Source: CAD feature listing. Evaluate the final solid. Frame: model axes, mm. Round coordinates to 2 decimals unless told otherwise and drop trailing zeros. Write each loop counter-clockwise with the first axis right and the second up, starting at its lowest first coordinate (ties: lowest second). Pieces come first, ordered by that corner, then holes.
from build123d import *

# Parameters (mm, degrees)
BOSS_EXTRUDE1_DEPTH = 3.175
SKETCH2_W           = 2.286
SKETCH2_H           = 69.616100292
BOSS_EXTRUDE2_DEPTH = 3.175
FILLET1_R           = 1


with BuildPart() as part:
    # Sketch1 → Boss-Extrude1 (new body)
    with BuildSketch(Plane(origin=(0, 0, 0), x_dir=(1, 0, 0), z_dir=(0, 1, 0))):
        Polygon((83.6803, 0), (96.3803, 0), (96.3803, 143.6878), (0, 143.6878), (0, 0), (12.7, 0), (12.7, -2.286), (83.6803, -2.286), align=None)
    extrude(amount=BOSS_EXTRUDE1_DEPTH)

    # Sketch2 → Boss-Extrude2 (add, through all)
    with BuildSketch(Plane.XZ):
        with Locations((-1.143, -87.286990146)):
            Rectangle(SKETCH2_W, SKETCH2_H)
        with Locations((97.5233, -87.286990146)):
            Rectangle(SKETCH2_W, SKETCH2_H)
    extrude(amount=-BOSS_EXTRUDE2_DEPTH)

    # Fillet1
    fillet1_edges = [part.edges().sort_by_distance(p)[0] for p in [
        (0, 1.5875, -143.6878),
        (96.3803, 1.5875, -143.6878),
        (96.3803, 1.5875, 0),
        (83.6803, 1.5875, 2.286),
        (12.7, 1.5875, 2.286),
        (0, 1.5875, 0),
        (0, 1.5875, -52.47894),
        (0, 1.5875, -122.095040292),
        (-2.286, 1.5875, -122.095040292),
        (-2.286, 1.5875, -52.47894),
        (96.3803, 1.5875, -122.095040292),
        (96.3803, 1.5875, -52.47894),
        (98.6663, 1.5875, -52.47894),
        (98.6663, 1.5875, -122.095040292),
    ]]
    fillet(fillet1_edges, radius=FILLET1_R)


solid = part.part
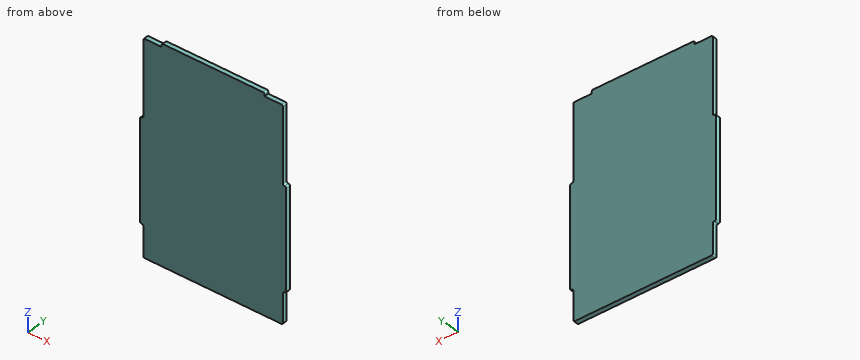
1) Material intervals for line 1 (X direction, y = 2.3, z = -50.5); line 2 (Z direction, x = 90, y = 2.3), sorted ascending.
Taken from the geometry:
line 1: x = 0 to 96.38
line 2: z = -143.69 to 0
2) Contact query for flat-ended pins moving along their axis: P1, Ø1.4, axis at y = 1.5, z = 0.5, coming from the -X side; P2, Ø1, axis at x = 6.5, y = 1.5, coming from the +Z side; P3, Ø0.6, axis at y = 2, z = 0.5, coming from the +X side. Output: stop coordinate, or through.
Taken from the geometry:
P1: stops at x = 0.4
P2: stops at z = 0
P3: stops at x = 83.68
3) Section query C-C on x = 92. Return the cut outline in (y, z) (3 decimals).
Taken from the geometry:
outline: (0, -143.688) - (3.175, -143.688) - (3.175, 0) - (0, 0) - close
4) Section query B-B on z = -31. Return the cut outline in (x, y) (3 decimals), then the cut area to 3 significant figures.
Taken from the geometry:
outline: (0, 0) - (96.38, 0) - (96.38, 3.175) - (0, 3.175) - close
area: 306 mm2
